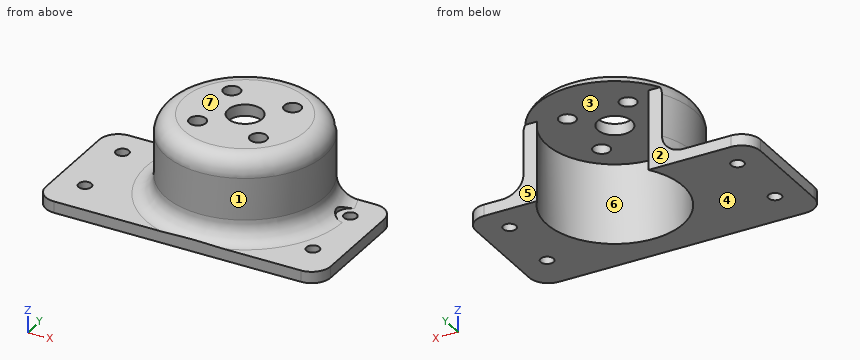
Autodesk Inventor part; units mm, degrees
ref_plane "Work Plane1" through (-53.798179, 52.016597, 21) normal (0, 0, 1) x (0.817541, 0.5758704, 0)
ref_plane "YZ Plane" through (0, 0, 0) normal (1, 0, 0) x (0, 1, 0)
ref_plane "XZ Plane" through (0, 0, 0) normal (0, 1, 0) x (-1, 0, 0)
sketch "Sketch1" plane through (0, 0, 0) normal (0, 0, 1) x (1, 0, 0)
  circle A0 centre (-15, 75) radius 1.7
  circle A1 centre (-15, 57.5) radius 1.7
  circle A2 centre (-75, 75) radius 1.7
  circle A3 centre (-75, 57.5) radius 1.7
  line L0 (-67.5, 62.5) -> (-67.5, 82.5)
  arc A4 (-67.5, 62.5) -> (-57.5, 52.5) centre (-57.5, 62.5) ccw
  line L1 (-32.5, 52.5) -> (-57.5, 52.5)
  arc A5 (-32.5, 52.5) -> (-22.5, 62.5) centre (-32.5, 62.5) ccw
  line L2 (-22.5, 82.5) -> (-22.5, 62.5)
  line L3 (-7.5, 82.5) -> (-22.5, 82.5)
  line L4 (-7.5, 62.5) -> (-7.5, 82.5)
  line L5 (-67.5, 82.5) -> (-82.5, 82.5)
  line L6 (-82.5, 82.5) -> (-82.5, -37.5)
  line L7 (-82.5, 52.5) -> (-57.5, 52.5)
  line L8 (-32.5, 52.5) -> (-7.5, 52.5)
  line L9 (-7.5, 52.5) -> (-7.5, 62.5)
  circle A6 centre (-41.087567, 72.129389) radius 17.98
  line L10 (-67.5, 82.5) -> (-55.775345, 82.5)
  line L11 (-22.5, 82.5) -> (-26.399789, 82.5)
  line L12 (-7.5, 52.5) -> (-82.5, 52.5)
  line L13 (-82.5, 52.5) -> (-82.5, 47.5)
  line L14 (-82.5, 47.5) -> (-7.5, 47.5)
  line L15 (-7.5, 47.5) -> (-7.5, 52.5)
  point P0 (0, 0)
  point P1 (-22.296102, 67.952867)
  dimension "d2" = 5
extrude "Extrusion1" add sketch "Sketch1" along normal blind 3 contours A4 L7 L6 L5 L0 | L0 L10 A6 L11 L2 A5 L1 A4 | L1 L8 L15 L14 L6 L7 | A5 L2 L3 L4 L9 L8
sketch "Sketch2" plane through (0, 0, 3) normal (0, 0, 1) x (1, 0, 0)
  circle A0 centre (-41.087567, 72.129389) radius 17.98
  line L0 (-55.775345, 82.5) -> (-82.5, 82.5)
  line L1 (-7.5, 82.5) -> (-26.399789, 82.5)
  circle A1 centre (-41.087567, 72.129389) radius 20.98
  point P0 (0, 0)
  point P1 (-59.325188, 82.5)
  point P2 (-22.849946, 82.5)
  dimension "d3" = 3
ref_plane "Work Plane1" through (-53.798179, 52.016597, 21) normal (0, 0, 1) x (0.817541, 0.5758704, 0)
extrude "Extrusion2" add sketch "Sketch2" along normal up to surface (18 mm away) contours A0 L1 A1 L0 picked at (-21.478975, 69.046328)
sketch "Sketch3" plane through (-41.087567, 72.129389, 21) normal (0, 0, 1) x (1, 0, 0)
  arc A0 (-18.237621, 10.370611) -> (18.237621, 10.370611) centre (0, 0) ccw
  circle A1 centre (0, 0) radius 4.485
  arc A2 (-14.687778, 10.370611) -> (14.687778, 10.370611) centre (0, 0) ccw construction
  line L0 (0, 0) -> (11.25, 0) construction
  line L1 (8, 0) -> (8, -8) construction
  line L2 (0, 0) -> (0, -11.25) construction
  circle A3 centre (8, -8) radius 2.2
  circle A4 centre (-8, -8) radius 2.2
  circle A5 centre (0, 0) radius 20.98
  circle A6 centre (8, 8) radius 2.2
  circle A7 centre (-8, 8) radius 2.2
  point P0 (41.087567, -72.129389)
  point P1 (18.237621, 10.370611)
  point P2 (-18.237621, 10.370611)
  dimension "d6" = 8
  dimension "d7" = 4.4
  dimension "d20" = 16
  dimension "d21" = 8
extrude "Extrusion3" add sketch "Sketch3" along normal blind 3
fillet "Fillet1" radius 5 4 edges at (-82.5, 82.5, 1.5) (-82.5, 47.5, 1.5) (-7.5, 47.5, 1.5) (-7.5, 82.5, 1.5)
fillet "Fillet2" radius 5 1 edges at (-41.0876, 51.1494, 3)
fillet "Fillet3" radius 5 1 edges at (-59.3252, 61.7588, 24)
sketch "Sketch4" plane through (0, 0, 3) normal (0, 0, 1) x (1, 0, 0)
  circle A0 centre (-15, 57.5) radius 1.7
  arc A1 (-15.134193, 73.305305) -> (-15.499481, 76.624967) centre (-15, 75) ccw
  circle A2 centre (-75, 75) radius 1.7
  circle A3 centre (-75, 57.5) radius 1.7
  circle A4 centre (-15, 57.5) radius 3.5
  circle A5 centre (-75, 57.5) radius 3.5
  circle A6 centre (-75, 75) radius 3.5
  circle A7 centre (-15, 75) radius 1.7
  circle A8 centre (-15, 75) radius 3.5
  point P0 (0, 0)
  dimension "d13" = 7
  dimension "d14" = 7
  dimension "d15" = 7
  dimension "d16" = 7
extrude "Extrusion4" cut sketch "Sketch4" along normal blind 3
properties part number "Rex Motor Bracket"
The listing builds one solid part. Answer for the finished solid, in the listing's coordinates (mm). Face numbers are marked on the shaded views. A direction names the side the tool comes from. Give positions to 0.01 mm unless a question says otherwise; leave off trailing zeros. Order: outer loops, then holes, each group sorted by start corner. A loop starts at its lowest first (then second) coordinate and runs counter-clockwise, first axis right, second up. Notation, with made-up numbers: (40.5, 85) -> (98.5, 85) arc R24 ccw to (98.5, 104) -> close; hole circle Ø2 at (35.5, 34.5). An arc over 180 degrees is marked (long way). Answer as a JSON object with one key per item and string values. Group by question number.
Item 1: Flat-ended cylindrical pins translate along their axes: pin 1 (10 mm diameter, centred on x = -36, z = 12, fed in from -Y); pin 2 (1 mm diameter, centred on x = -31, y = 87.5, fed in from +Z); pin 3 (12 mm diameter, centred on y = 67, z = 15.5, fed in from -X). Find the tip coordinate at first contact, or state that the pin passes through.
Item 2: The part is cut by section B-B on z = 2.25. Write down the section's boundary in (x, y).
Item 3: The part is cut by section C-C on y = 57.5. Give the number of separate pieces and of enclosed holes in the cut face, and give its area (3 significant figures).
Item 4: Determine the mould class of the marked faces 5, 6 and 7 for opening direction Y: pulls with the +Y half, pulls with the -Y half, needs draft (parallel to the pull), parting line crosses it, or undercut.
Item 5: A tool of negligible diameter and unlimited length cuts with its end or side. For the marked faces 1, 2, 3 and 4, from which of +Z, -Z, +X, -X, +Y, -Y can it reach the whole face along a straight path? Write none if from no direction.
Item 6: The part is cut by section A-A on x = -75. Write down the section's boundary in (y, z), and give its area (3 significant figures).
Item 7: Consider L1, parallel to Y at x = -15, z = 0.8; L2, parallel to X at y = 75, z = 1.05; L3, parallel to Z at x = -71, y = 62. Determine where each line is inside the solid, lowest interval first. Write a range as from..to.
Item 8: The part is cut by section D-D on z = 16.75. Write down the section's boundary in (x, y).
Result set:
{
 "1": {"pin 1": "y = 51.15", "pin 2": "z = 23.62", "pin 3": "x = -62.07"},
 "2": {"outline": "(-82.5, 52.5) arc R5 ccw to (-77.5, 47.5) -> (-12.5, 47.5) arc R5 ccw to (-7.5, 52.5) -> (-7.5, 77.5) arc R5 ccw to (-12.5, 82.5) -> (-26.4, 82.5) arc R17.98 cw (long way) to (-55.78, 82.5) -> (-77.5, 82.5) arc R5 ccw to (-82.5, 77.5) -> close; hole circle Ø3.4 at (-75, 57.5); hole circle Ø3.4 at (-75, 75); hole circle Ø3.4 at (-15, 57.5); hole circle Ø3.4 at (-15, 75)"},
 "3": {"separate pieces": "3", "enclosed holes": "0", "area": "396 mm²"},
 "4": {"face 5": "pulls with the +Y half", "face 6": "undercut", "face 7": "needs draft"},
 "5": {"face 1": "+Z", "face 2": "-Z, +X, -X, +Y", "face 3": "-Z", "face 4": "-Z, +X, -X, +Y, -Y"},
 "6": {"outline": "(47.5, 0) -> (55.8, 0) -> (55.8, 3) -> (47.5, 3) -> close; (59.2, 0) -> (73.3, 0) -> (73.3, 3) -> (59.2, 3) -> close; (76.7, 0) -> (82.5, 0) -> (82.5, 3) -> (76.7, 3) -> close", "area": "84.6 mm²"},
 "7": {"L1": "47.5..55.8, 59.2..73.3, 76.7..82.5", "L2": "-82.5..-76.7, -73.3..-58.84, -23.34..-16.7, -13.3..-7.5", "L3": "0..3"},
 "8": {"outline": "(-59.33, 82.5) arc R20.98 ccw (long way) to (-22.85, 82.5) -> (-26.4, 82.5) arc R17.98 cw (long way) to (-55.78, 82.5) -> close"}
}
